The model under review builds one solid part; all positions refer to its coordinate system, in mm. A direction names the side the tool comes from. Give positions to 0.01 mm unless a question says otherwise; leave off trailing zeros. Order: outer loops, then holes, each group sorted by start corner. A loop starts at its lowest first (then second) coordinate and runs counter-clockwise, first axis right, second up. Notation, with made-up numbers: (32.25, 72.25) - (71.25, 72.25) arc R19 ccw to (71.25, 97.25) - close; hole circle Ø7 at (44.5, 79.5). An arc over 180 degrees is marked (long way). Use CSV: the item, a comma, the result in double quotes. Start each with the question number.
```python
from build123d import *

# Parameters (mm, degrees)
SKETCH1_W           = 185
SKETCH1_H           = 120
BOSS_EXTRUDE1_DEPTH = 10
BOSS_EXTRUDE2_DEPTH = 14
BOSS_EXTRUDE3_DEPTH = 157
BOSS_EXTRUDE4_DEPTH = 14
SKETCH6_W           = 120
SKETCH6_H           = 10
CUT_EXTRUDE1_DEPTH  = 300
SKETCH7_W           = 15
SKETCH7_H           = 94
BOSS_EXTRUDE5_DEPTH = 10
SKETCH8_R           = 1
CUT_EXTRUDE2_DEPTH  = 4
SKETCH9_R           = 1
CUT_EXTRUDE3_DEPTH  = 4
FILLET1_R           = 5
SKETCH10_W          = 8.94
SKETCH10_H          = 3.16
CUT_EXTRUDE4_DEPTH  = 13
FILLET2_R           = 1
SKETCH12_W          = 18.3
SKETCH12_H          = 2
CUT_EXTRUDE6_DEPTH  = 13
SKETCH13_W          = 18.3
SKETCH13_H          = 2
BOSS_EXTRUDE6_DEPTH = 7.89


with BuildPart() as part:
    # Sketch1 → Boss-Extrude1 (new body)
    with BuildSketch(Plane(origin=(0, 0, 0), x_dir=(1, 0, 0), z_dir=(0, 1, 0))):
        Rectangle(SKETCH1_W, SKETCH1_H)
    extrude(amount=BOSS_EXTRUDE1_DEPTH)

    # Sketch3 → Boss-Extrude2 (add)
    with BuildSketch(Plane(origin=(92.5, 0, 0), x_dir=(0, 0, -1), z_dir=(1, 0, 0))):
        Polygon((60, 0), (-35.195789495, -86.829236424), (-60, 0), align=None)
    extrude(amount=-BOSS_EXTRUDE2_DEPTH)

    # Sketch4 → Boss-Extrude3 (add)
    with BuildSketch(Plane.ZY.offset(-78.5)):
        Polygon((35.141852327, -39.693461507), (47, 0), (60, 0), (35.195789495, -86.829236424), (-60, 0), (-47, 0), (-4.415483527, -33.157236801), (31.435973084, -61.614600076), align=None)
    extrude(amount=BOSS_EXTRUDE3_DEPTH)

    # Sketch5 → Boss-Extrude4 (add)
    with BuildSketch(Plane.ZY.offset(78.5)):
        Polygon((60, 0), (-60, 0), (35.195789495, -86.829236424), align=None)
    extrude(amount=BOSS_EXTRUDE4_DEPTH)

    # Sketch6 → Cut-Extrude1 (cut)
    with BuildSketch(Plane.ZY.offset(92.5)):
        with Locations((0, 5)):
            Rectangle(SKETCH6_W, SKETCH6_H)
    extrude(amount=-CUT_EXTRUDE1_DEPTH, mode=Mode.SUBTRACT)

    # Sketch7 → Boss-Extrude5 (add)
    with BuildSketch(Plane(origin=(0, 0, 0), x_dir=(1, 0, 0), z_dir=(0, 1, 0))):
        with Locations((6.531892019, 0)):
            Rectangle(SKETCH7_W, SKETCH7_H)
    extrude(amount=-BOSS_EXTRUDE5_DEPTH)

    # Sketch8 → Cut-Extrude2 (cut)
    with BuildSketch(Plane(origin=(0, 0, 0), x_dir=(1, 0, 0), z_dir=(0, 1, 0))):
        with Locations((87.5, -55)):
            Circle(SKETCH8_R)
        with Locations((-87.5, -55)):
            Circle(SKETCH8_R)
        with Locations((12.5, -55)):
            Circle(SKETCH8_R)
        with Locations((2.5, -55)):
            Circle(SKETCH8_R)
    extrude(amount=-CUT_EXTRUDE2_DEPTH, mode=Mode.SUBTRACT)

    # Sketch9 → Cut-Extrude3 (cut)
    with BuildSketch(Plane(origin=(0, 0, 0), x_dir=(1, 0, 0), z_dir=(0, 1, 0))):
        with Locations((87.5, 50)):
            Circle(SKETCH9_R)
        with Locations((-87.5, 50)):
            Circle(SKETCH9_R)
        with Locations((12.5, 50)):
            Circle(SKETCH9_R)
        with Locations((2.5, 50)):
            Circle(SKETCH9_R)
    extrude(amount=-CUT_EXTRUDE3_DEPTH, mode=Mode.SUBTRACT)

    # Fillet1
    fillet1_edges = [part.edges().sort_by_distance(p)[0] for p in [
        (0, -86.829236424, 35.195789495),
    ]]
    fillet(fillet1_edges, radius=FILLET1_R)

    # Sketch10 → Cut-Extrude4 (cut)
    with BuildSketch(Plane(origin=(0, -15.846809365, 55.473096258), x_dir=(1, 0, 0), z_dir=(0, -0.274678714, 0.961536065))):
        with Locations((0, -18.026592613)):
            Rectangle(SKETCH10_W, SKETCH10_H)
    extrude(amount=-CUT_EXTRUDE4_DEPTH, mode=Mode.SUBTRACT)

    # Fillet2
    fillet2_edges = [part.edges().sort_by_distance(p)[0] for p in [
        (4.47, -29.895487229, 44.775936137),
        (4.47, -32.92871232, 43.889647284),
        (-4.47, -32.92871232, 43.889647284),
        (-4.47, -29.895487229, 44.775936137),
    ]]
    fillet(fillet2_edges, radius=FILLET2_R)

    # Sketch12 → Cut-Extrude6 (cut)
    with BuildSketch(Plane(origin=(0, -15.846809365, 55.473096258), x_dir=(1, 0, 0), z_dir=(0, -0.274678714, 0.961536065))):
        with Locations((0, -20.606592613)):
            Rectangle(SKETCH12_W, SKETCH12_H)
    extrude(amount=-CUT_EXTRUDE6_DEPTH, mode=Mode.SUBTRACT)

    # Sketch13 → Boss-Extrude6 (add)
    with BuildSketch(Plane(origin=(0, -15.846809365, 55.473096258), x_dir=(1, 0, 0), z_dir=(0, -0.274678714, 0.961536065))):
        with Locations((0, -20.606592613)):
            Rectangle(SKETCH13_W, SKETCH13_H)
    extrude(amount=-BOSS_EXTRUDE6_DEPTH)


solid = part.part
```
1. Consider section B-B (y = -17.5). Give the boundary of the cut face in (x, z).
2. Consider section C-C (x = 23.5). Give the boundary of the cut face in (y, z), and give its area (3 significant figures).
3. Consider section A-A (z = 8.5). Give the boundary of the cut face in (x, y), and give its area (3 significant figures).
4. Tool access review of faces 4 (the face through (-78.5, -24, 10)), 5 (the face through (-0.05, -33.63, 46.35)), 6 (the face through (-4.47, -31, 44)), 7 (the face through (-1, 0, 52)): name each direction out of +Z, -Z, +X, -X, +Y, -Y from which nothing blocks a thin tool from reaching the whole face with its end or side.
5. Clearance check with flat-ended pins moving along their axes: pin 1 (1.8 mm diameter, centred on x = 12.5, z = -50, fed in from +Y); pin 2 (1 mm diameter, centred on x = 13, z = -49.5, fed in from +Y); pin 3 (10 mm diameter, centred on x = -28.5, z = -24.5, fed in from -Y); pin 4 (10 mm diameter, centred on x = -14, y = -69, fed in from +Z). State where each tip first meets the part, or that it passes through.
6. To check wall thickness, follow L1, parallel to X at y = -3, z = 55; L2, parallel to X at y = -53.5, z = 31; L3, parallel to Z at x = -87.5, y = -0.9. State the ranges of each line that lie inside material, in increasing order. Write a range as [from, to].
7. Mouldability with a two-part tool opening along X and no side actions: class faces 1 (the face through (-92.5, -32, 12)), 2 (the face through (-6.35, -31.855, 40.13)), 3 (the face through (-1.295, -82.527, 33.901)) as pulls with the +X half, pulls with the -X half, needs draft (parallel to the pull), parting line crosses it, or undercut.
8. Consider section D-D (y = -54.5). Give the boundary of the cut face in (x, z).
Answers follow:
1,outline,"(-92.5, -40.81) - (92.5, -40.81) - (92.5, 55) - (-92.5, 55) - close; hole (-78.5, -24.52) - (78.5, -24.52) - (78.5, 41.77) - (-78.5, 41.77) - close"
2,outline,"(-81.39, 29.23) - (0, -60) - (0, -47) - (-33.16, -4.42) - (-61.61, 31.44) - (-39.69, 35.14) - (0, 47) - (0, 60) - (-79.07, 37.41) arc R5 ccw to start"
2,area,"2,370 mm^2"
3,outline,"(-92.5, -62.48) - (92.5, -62.48) - (92.5, 0) - (78.5, 0) - (78.5, -43.41) - (-78.5, -43.41) - (-78.5, 0) - (-92.5, 0) - close; (-0.97, -10) - (14.03, -10) - (14.03, 0) - (-0.97, 0) - close"
3,area,"4,890 mm^2"
4,face 4,"+Y"
4,face 5,"+Z"
4,face 6,"none"
4,face 7,"+Z, -Z, +X, -X, +Y"
5,pin 1,"stops at y = -4"
5,pin 2,"stops at y = 0"
5,pin 3,"stops at y = -36.94"
5,pin 4,"stops at z = 41.72"
6,L1,"x = [-92.5, -88.5], [-86.5, 1.5], [3.5, 11.5], [13.5, 86.5], [88.5, 92.5]"
6,L2,"x = [-92.5, -78.5], [78.5, 92.5]"
6,L3,"z = [-59.01, -51], [-49, 54], [56, 59.74]"
7,face 1,"pulls with the -X half"
7,face 2,"undercut"
7,face 3,"needs draft"
8,outline,"(-92.5, -0.25) - (92.5, -0.25) - (92.5, 44.43) - (-92.5, 44.43) - close; hole (-78.5, 22.47) - (78.5, 22.47) - (78.5, 32.64) - (-78.5, 32.64) - close"
